Read the model definition and answer for the solid it produces. Units are mm, in the model's axes. A direction names the side the tool comes from. Round coordinates to 2 decimals unless told otherwise and drop trailing zeros. Write each loop counter-clockwise with the first axis right and the second up, starting at its lowest first coordinate (ties: lowest second). Pieces come first, ordered by that corner, then holes. Notation, with made-up numbers: (59.5, 54.5) -> (111.5, 54.5) arc R4 cw to (111.5, 61.5) -> close; hole circle Ø3 at (-16, 86). An arc over 180 degrees is marked (long way). Return JSON: item names as keys, results as strings. Group by question number.
(1) A cutting plane is placed at B-B on x = 8.5. Give the vertices of the cut face in (y, z), then the cut area to 3 significant figures.
(2) A cutting plane is placed at C-C on y = 4.75. State how many separate pieces and enclosed holes the cut face has, then the cut area to 3 significant figures.
(3) Given pin 1 (1 mm diameter, centred on x = 0.5, y = 9, fed in from +Z); pin 2 (2 mm diameter, centred on x = -8, y = 4.5, fed in from -Z); pin 3 (0.7 mm diameter, centred on x = 3.5, z = 13.5, fed in from +Y), each flat-ended and moving along its own axis, determine where each tip first touches the part or whether it passes through.
(4) For faces 1 (the flat face through (6, 5, -13.958)), 2 (the flat face through (-1.429, 5, -11)), 3 (the flat face through (4, 3, 12.037)), 4 (the flat face through (2.019, 3, -1)), 5 (the flat face through (0.854, 7, -10)), determine the directions among +Z, -Z, +X, -X, +Y, -Y from which every point of the face is accessible in a straight line to the end or side of a thin tool.
(5) The mould has two halves that part along Y. Classify faces 6 (the flat face through (5.784, 9.775, -13.374)), 7 (the flat face through (-8, 2.02, -11)), 8 (the flat face through (8.009, 3, -1)): released by +Y, released by -Y, zero draft, split by the parting line, or undercut.
(6) A cutting plane is placed at A-A on y = 11.25. Give the vertices of the cut face in (x, z).
(7) Straight lines are drawn through the part: line 1 (Z direction, x = 7, y = 3.5); line 2 (Z direction, x = 3.75, y = 3.75); line 3 (Z direction, x = 1, y = 6.75). For each, find the intervals that lie inside material, in ascending order.
```python
from build123d import *

# Parameters (mm, degrees)
SKETCH_1_W              = 23.3
SKETCH_1_H              = 29.2
EXTRUDE_1_DEPTH         = 1.6
EXTRUDE_2_DEPTH         = 2.54
SKETCH_3_W              = 0.6
SKETCH_3_H              = 0.6
EXTRUDE_3_DEPTH         = 6
PATTERN_LINEAR_11_COUNT = 6
PATTERN_LINEAR_11_PITCH = 2.54
SKETCH_4_W              = 6.084765078
SKETCH_4_H              = 4.622534711
SKETCH_4_W_2            = 5.990427635
EXTRUDE_4_DEPTH         = 2
SKETCH_5_W              = 10
SKETCH_5_H              = 7.86
EXTRUDE_5_DEPTH         = 10
CUT_EXTRUDE_1_DEPTH     = 28
SKETCH_7_W              = 4.089618495
SKETCH_7_H              = 5.460987571
CUT_EXTRUDE_2_DEPTH     = 6
SKETCH_8_R              = 1.55
SKETCH_8_W              = 0.408344746
SKETCH_8_H              = 3.212311997
CUT_EXTRUDE_3_DEPTH     = 6


with BuildPart() as part:
    # 草图1 → 凸台-拉伸1 (new body)
    with BuildSketch(Plane(origin=(0, 0, 0), x_dir=(1, 0, 0), z_dir=(0, 1, 0))):
        Rectangle(SKETCH_1_W, SKETCH_1_H)
    extrude(amount=EXTRUDE_1_DEPTH)

    # 草图2 → 凸台-拉伸2 (add)
    with BuildSketch(Plane(origin=(0, 1.6, 0), x_dir=(1, 0, 0), z_dir=(0, 1, 0))):
        Polygon((-4.668338696, -12.037397235), (-2.959469598, -12.037397235), (-2.535205529, -12.461661304), (-2.110941461, -12.037397235), (-0.402072363, -12.037397235), (0.022191706, -12.461661304), (0.446455775, -12.037397235), (2.155324873, -12.037397235), (2.579588942, -12.461661304), (3.00385301, -12.037397235), (4.712722108, -12.037397235), (5.136986177, -12.461661304), (5.561250246, -12.037397235), (7.270119344, -12.037397235), (7.694383412, -12.461661304), (7.694383412, -14.178338696), (7.270119344, -14.602602765), (5.561250246, -14.602602765), (5.136986177, -14.178338696), (4.712722108, -14.602602765), (3.00385301, -14.602602765), (2.579588942, -14.178338696), (2.155324873, -14.602602765), (0.446455775, -14.602602765), (0.022191706, -14.178338696), (-0.402072363, -14.602602765), (-2.110941461, -14.602602765), (-2.535205529, -14.178338696), (-2.959469598, -14.602602765), (-4.668338696, -14.602602765), (-5.092602765, -14.178338696), (-5.516866833, -14.602602765), (-7.225735931, -14.602602765), (-7.65, -14.178338696), (-7.65, -12.461661304), (-7.225735931, -12.037397235), (-5.516866833, -12.037397235), (-5.092602765, -12.461661304), align=None)
    extrude(amount=EXTRUDE_2_DEPTH)

    # 草图3 → 凸台-拉伸3 (add)
    with BuildSketch(Plane(origin=(0, 4.14, 0), x_dir=(1, 0, 0), z_dir=(0, 1, 0))):
        with Locations((-6.371301382, -13.32)):
            Rectangle(SKETCH_3_W, SKETCH_3_H)
    extrude_3 = extrude(amount=EXTRUDE_3_DEPTH)

    # 阵列(线性)11: 凸台-拉伸3 ×6
    with Locations(*[(i * PATTERN_LINEAR_11_PITCH, 0, 0) for i in range(1, PATTERN_LINEAR_11_COUNT)]):
        add(extrude_3)

    # 草图4 → 凸台-拉伸4 (add)
    with BuildSketch(Plane(origin=(0, 1.6, 0), x_dir=(1, 0, 0), z_dir=(0, 1, 0))):
        with Locations((-4.891303326, 1.247938362)):
            Rectangle(SKETCH_4_W, SKETCH_4_H)
        with Locations((5.014128197, 1.247938362)):
            Rectangle(SKETCH_4_W_2, SKETCH_4_H)
    extrude(amount=EXTRUDE_4_DEPTH)

    # 草图5 → 凸台-拉伸5 (add)
    with BuildSketch(Plane(origin=(0, 1.6, 0), x_dir=(1, 0, 0), z_dir=(0, 1, 0))):
        with Locations((-5.85390251, 10.028478066)):
            Rectangle(SKETCH_5_W, SKETCH_5_H)
        with Locations((5.85390251, 10.028478066)):
            Rectangle(SKETCH_5_W, SKETCH_5_H)
    extrude(amount=EXTRUDE_5_DEPTH)

    # 草图6 → 切除-拉伸1 (cut)
    with BuildSketch(Plane.ZY.offset(10.85390251)):
        Polygon((-13.958478066, 8), (-12.773407339, 11.6), (-7.773407339, 11.6), (-6.098478066, 8), (-4.60674586, 8), (-4.60674586, 12.734862091), (-15.29251654, 12.734862091), (-15.29251654, 8), align=None)
    extrude(amount=-CUT_EXTRUDE_1_DEPTH, mode=Mode.SUBTRACT)

    # 草图7 → 切除-拉伸2 (cut)
    with BuildSketch(Plane(origin=(0, 0, -13.958478066), x_dir=(-1, 0, 0), z_dir=(0, 0, -1))):
        with Locations((-8.248950011, 4.75004571)):
            Rectangle(SKETCH_7_W, SKETCH_7_H)
        with Locations((8.248950011, 4.75004571)):
            Rectangle(SKETCH_7_W, SKETCH_7_H)
        with Locations((3.473646978, 4.75004571)):
            Rectangle(SKETCH_7_W, SKETCH_7_H)
        with Locations((-3.473646978, 4.75004571)):
            Rectangle(SKETCH_7_W, SKETCH_7_H)
    extrude(amount=-CUT_EXTRUDE_2_DEPTH, mode=Mode.SUBTRACT)

    # 草图8 → 切除-拉伸3 (cut)
    with BuildSketch(Plane(origin=(0, 11.6, 0), x_dir=(1, 0, 0), z_dir=(0, 1, 0))):
        with Locations(Location((-8.35390251, 10.273407339, 0), (0, 0, 270))):
            Circle(SKETCH_8_R)
        with Locations(Location((-3.35390251, 10.273407339, 0), (0, 0, 270))):
            Circle(SKETCH_8_R)
        with Locations(Location((8.35390251, 10.273407339, 0), (0, 0, 180))):
            Circle(SKETCH_8_R)
        with Locations(Location((3.35390251, 10.273407339, 0), (0, 0, 180))):
            Circle(SKETCH_8_R)
        with Locations((-5.919084565, 10.231849543)):
            Rectangle(SKETCH_8_W, SKETCH_8_H)
        with Locations((5.919084565, 10.231849543)):
            Rectangle(SKETCH_8_W, SKETCH_8_H)
    extrude(amount=-CUT_EXTRUDE_3_DEPTH, mode=Mode.SUBTRACT)


solid = part.part
```
Checks:
{
 "1": {"outline": "(0, -14.6) -> (1.6, -14.6) -> (1.6, -13.96) -> (2.02, -13.96) -> (2.02, -7.96) -> (7.48, -7.96) -> (7.48, -8.73) -> (11.6, -8.73) -> (11.6, -7.77) -> (8, -6.1) -> (1.6, -6.1) -> (1.6, 14.6) -> (0, 14.6) -> close; (7.48, -13.96) -> (8, -13.96) -> (11.6, -12.77) -> (11.6, -11.82) -> (7.48, -11.82) -> close", "area": "74.7 mm^2"},
 "2": {"separate pieces": "8", "enclosed holes": "0", "area": "61.2 mm^2"},
 "3": {"pin 1": "stops at z = 13.62", "pin 2": "stops at z = -7.96", "pin 3": "stops at y = 10.14"},
 "4": {"face 1": "-Z, +X, -X, +Y", "face 2": "-Z", "face 3": "+X, -X, +Y", "face 4": "+Y", "face 5": "-Z, +Y"},
 "5": {"face 6": "released by +Y", "face 7": "undercut", "face 8": "zero draft"},
 "6": {"outline": "(-10.85, -12.89) -> (-0.85, -12.89) -> (-0.85, -7.61) -> (-10.85, -7.61) -> close; (0.85, -12.89) -> (10.85, -12.89) -> (10.85, -7.61) -> (0.85, -7.61) -> close; hole circle Ø3.1 at (-8.35, -10.27); hole (-6.12, -11.84) -> (-5.71, -11.84) -> (-5.71, -8.63) -> (-6.12, -8.63) -> close; hole circle Ø3.1 at (-3.35, -10.27); hole circle Ø3.1 at (3.35, -10.27); hole (5.71, -11.84) -> (6.12, -11.84) -> (6.12, -8.63) -> (5.71, -8.63) -> close; hole circle Ø3.1 at (8.35, -10.27)"},
 "7": {"line 1": "z = -7.96 to -6.1, -3.56 to 1.06, 12.04 to 14.6", "line 2": "z = -7.96 to -6.1, 12.04 to 14.6", "line 3": "z = -13.96 to -6.1, 13.02 to 13.62"}
}
